For this review, take the finished solid that the model builds, in its own axes (mm). Face numbers are marked on the shaded views. A direction names the side the tool comes from. Round coordinates to 2 decimals unless told otherwise and drop trailing zeros. Order: outer loops, then holes, each group sorted by start corner. A loop starts at its lowest first (then second) coordinate and runs counter-clockwise, first axis right, second up. Notation, with made-up numbers: (-26, 58.5) -> (5, 58.5) arc R31 cw to (5, 93.5) -> close; hole circle Ø7 at (85, 8.25). An arc over 180 degrees is marked (long way). Answer in a Markdown table with one row per item.
```python
from build123d import *

# Parameters (mm, degrees)
F0_W      = 25.4
F0_H      = 25.4
F1_DEPTH  = 25.4
F2_W      = 12.0143074892
F2_H      = 3.6042919382
F3_DEPTH  = 25.401
F4_W      = 3.3513596281
F4_H      = 17.4523624592
F5_DEPTH  = 25.401
F6_W      = 7.8409165144
F6_H      = 2.7822614647
F7_DEPTH  = 25.401
F10_W     = 12.962804758
F10_H     = 17.0729630627
F11_DEPTH = 25.401
F8_W      = 3.857224714
F8_H      = 2.5925613008
F12_DEPTH = 25.4
F9_W      = 4.8689562827
F9_H      = 2.6557944948
F13_DEPTH = 25.4
F15_W     = 0.9836773388
F15_H     = 3.4875846468
F16_DEPTH = 25.4
F17_W     = 0.9571057744
F17_H     = 4.5728415716
F18_DEPTH = 25.4


with BuildPart() as f1:
    # F0 (on Top) → F1 (new body)
    with BuildSketch(Plane.XY):
        with Locations((-0.6015789695, 2.4779321572)):
            Rectangle(F0_W, F0_H)
    extrude(amount=F1_DEPTH)

    # F2 (on face) → F3 (cut, through all)
    with BuildSketch(Plane.XY.offset(25.4)):
        with Locations((-6.5916299645, 12.428777758)):
            Rectangle(F2_W, F2_H)
    extrude(amount=-F3_DEPTH, mode=Mode.SUBTRACT)

    # F4 (on face) → F5 (cut, through all)
    with BuildSketch(Plane.XY.offset(25.4)):
        with Locations((-6.4967800863, 1.9004505593)):
            Rectangle(F4_W, F4_H)
    extrude(amount=-F5_DEPTH, mode=Mode.SUBTRACT)

    # F6 (on face) → F7 (cut, through all)
    with BuildSketch(Plane.XY.offset(25.4)):
        with Locations((-8.7415585294, -8.2168614026)):
            Rectangle(F6_W, F6_H)
    extrude(amount=-F7_DEPTH, mode=Mode.SUBTRACT)

    # F10 (on face) → F11 (cut, through all)
    with BuildSketch(Plane.XY.offset(25.4)):
        with Locations((4.852715123, 0.7451490965)):
            Rectangle(F10_W, F10_H)
    extrude(amount=-F11_DEPTH, mode=Mode.SUBTRACT)



with BuildPart() as f12:
    # F8 (on face) → F12 (new body)
    with BuildSketch(Plane.XY.offset(25.4)):
        with Locations((4.3793295044, 5.7260587346)):
            Rectangle(F8_W, F8_H)
    extrude(amount=-F12_DEPTH)


with BuildPart() as f13:
    # F9 (on face) → F13 (new body)
    with BuildSketch(Plane.XY.offset(25.4)):
        with Locations((5.4218145087, -3.2385426457)):
            Rectangle(F9_W, F9_H)
    extrude(amount=-F13_DEPTH)


with BuildPart() as f1_1:
    add(f1.part)

    add(f12.part)  # F16 merges F12
    # F15 (on face) → F16 (join)
    with BuildSketch(Plane.XY):
        with Locations((3.4799792338, 8.1227321643)):
            Rectangle(F15_W, F15_H)
    extrude(amount=F16_DEPTH)


    add(f13.part)  # F18 merges F13
    # F17 (on face) → F18 (join)
    with BuildSketch(Plane.XY):
        with Locations((5.6787764188, -6.1330919852)):
            Rectangle(F17_W, F17_H)
    extrude(amount=F18_DEPTH)


solid = f1_1.part
```
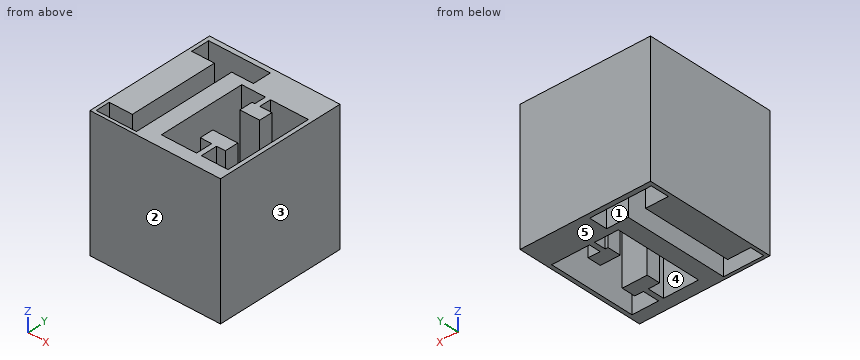
Q1. Take a section at C-C, the plane y = 5. Write out the cut boundary in (x, z).
Answer key:
| item | result |
|---|---|
| outline | (-13.3, 0) -> (-8.17, 0) -> (-8.17, 25.4) -> (-13.3, 25.4) -> close; (-4.82, 0) -> (-1.63, 0) -> (-1.63, 25.4) -> (-4.82, 25.4) -> close; (2.45, 0) -> (6.31, 0) -> (6.31, 25.4) -> (2.45, 25.4) -> close; (11.33, 0) -> (12.1, 0) -> (12.1, 25.4) -> (11.33, 25.4) -> close |
Q2. The part is to be moulded in two halves that separate along Y. For the marked faces 1, 2 and 3, say which applies: +Y half, -Y half, draft (parallel to the pull), parting line (faces both ways), or undercut.
Answer key:
| item | result |
|---|---|
| face 1 | undercut |
| face 2 | -Y half |
| face 3 | draft |
Q3. Take a section at D-D, the plane z = 15.25. Give the number of separate pieces and of enclosed holes in the cut face, then the cut area to 3 significant figures.
Answer key:
| item | result |
|---|---|
| separate pieces | 1 |
| enclosed holes | 2 |
| area | 328 mm^2 |
Q4. Take a section at B-B, the plane x = -7.75. Write out the cut boundary in (y, z), then the cut area to 3 significant figures.
Answer key:
| item | result |
|---|---|
| outline | (-10.22, 0) -> (-9.61, 0) -> (-9.61, 25.4) -> (-10.22, 25.4) -> close; (14.23, 0) -> (15.18, 0) -> (15.18, 25.4) -> (14.23, 25.4) -> close |
| area | 39.7 mm^2 |
Q5. To check wall thickness, follow probe 1 along X at (y, z) = (1.25, 15.75); probe 2 along Y at (x, z) = (7.25, 5.25); probe 3 along X at (y, z) = (-2, 8). State the ranges of each line that lie inside material, in increasing order.
Answer key:
| item | result |
|---|---|
| probe 1 | x = -13.3 to -8.17, -4.82 to -1.63, 11.33 to 12.1 |
| probe 2 | y = -10.22 to -7.79, -4.57 to -1.91, 9.28 to 15.18 |
| probe 3 | x = -13.3 to -8.17, -4.82 to -1.63, 2.99 to 7.86, 11.33 to 12.1 |
Q6. Tool access review of the marked faces 4 and 5: name each direction out of +Z, -Z, +X, -X, +Y, -Y from which nothing blocks a thin tool from reaching the whole face with its end or side.
Answer key:
| item | result |
|---|---|
| face 4 | +Z, -Z |
| face 5 | -Z, +X, -X, +Y, -Y |
Q7. Take a section at A-A, the plane y = 12.25. Write out the cut boundary in (x, z), then the cut area to 3 significant figures.
Answer key:
| item | result |
|---|---|
| outline | (-13.3, 0) -> (-12.6, 0) -> (-12.6, 25.4) -> (-13.3, 25.4) -> close; (-0.58, 0) -> (12.1, 0) -> (12.1, 25.4) -> (-0.58, 25.4) -> close |
| area | 340 mm^2 |
